Build history of the part. All positions in model axes, mm. Face numbers are marked on the shaded views. A direction names the side the tool comes from. Coordinates: 2 decimals unless noted, no trailing zeros. Order: outer loops, then holes, each group sorted by start corner. A loop starts at its lowest first (then second) coordinate and runs counter-clockwise, first axis right, second up. Notation, with made-up numbers: (87.25, 6.5) - (110.25, 6.5) arc R21 cw to (110.25, 22.5) - close; hole circle Ø11 at (-6, 79). An arc over 180 degrees is marked (long way). Return JSON: item names as keys, results as strings.
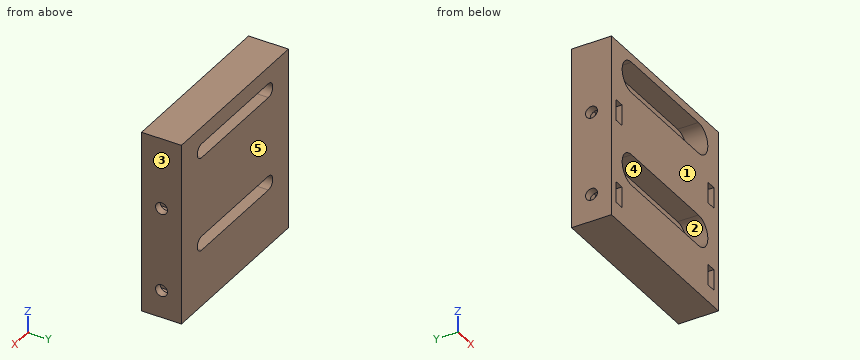
Autodesk Inventor part; units mm, degrees
ref_plane "YZ Plane" through (0, 0, 0) normal (1, 0, 0) x (0, 1, 0)
ref_plane "XZ Plane" through (0, 0, 0) normal (0, 1, 0) x (-1, 0, 0)
ref_plane "XY Plane" through (0, 0, 0) normal (0, 0, 1) x (1, 0, 0)
sketch "Sketch1" plane through (0, 0, 0) normal (0, 1, 0) x (-1, 0, 0)
  line L0 (-25.4, 20.32) -> (-25.4, -31.75)
  line L1 (-25.4, -31.75) -> (25.4, -31.75)
  line L2 (25.4, -31.75) -> (25.4, 20.32)
  line L3 (25.4, 31.75) -> (-25.4, -31.75) construction
  line L4 (-25.4, 31.75) -> (25.4, -31.75) construction
  line L5 (15.875, 13.4747) -> (-15.875, 13.4747) construction
  line L6 (15.875, 15.5067) -> (-15.875, 15.5067)
  line L7 (-15.875, 11.4427) -> (15.875, 11.4427)
  arc A0 (15.875, 11.4427) -> (15.875, 15.5067) centre (15.875, 13.4747) ccw
  arc A1 (-15.875, 15.5067) -> (-15.875, 11.4427) centre (-15.875, 13.4747) ccw
  line L8 (-15.875, -13.4747) -> (15.875, -13.4747) construction
  line L9 (-15.875, -15.5067) -> (15.875, -15.5067)
  line L10 (15.875, -11.4427) -> (-15.875, -11.4427)
  arc A2 (-15.875, -11.4427) -> (-15.875, -15.5067) centre (-15.875, -13.4747) ccw
  arc A3 (15.875, -15.5067) -> (15.875, -11.4427) centre (15.875, -13.4747) ccw
  line L11 (25.4, 20.32) -> (-25.4, 20.32)
  point P0 (0, 0)
  point P1 (0, 13.4747)
  point P2 (0, -13.4747)
  dimension "d0" = 50.8
  dimension "d2" = 26.9494
  dimension "d3" = 13.4747
  dimension "d4" = 26.9494
  dimension "d6" = 9.525
  dimension "d7" = 9.525
  dimension "d10" = 4.064
  dimension "d11" = 9.525
  dimension "d12" = 4.064
  dimension "d49" = 6.8453
extrude "Extrusion1" add sketch "Sketch1" along normal blind 11.43
sketch "Sketch3" plane through (0, 0, 0) normal (0, -1, 0) x (1, 0, 0)
  arc A0 (-15.875, -11.4427) -> (-15.875, -15.5067) centre (-15.875, -13.4747) ccw
  arc A1 (15.875, -15.5067) -> (15.875, -11.4427) centre (15.875, -13.4747) ccw
  line L0 (-15.875, -13.4747) -> (15.875, -13.4747) construction
  line L1 (-15.875, -17.9197) -> (15.875, -17.9197)
  line L2 (15.875, -9.0297) -> (-15.875, -9.0297)
  arc A2 (-15.875, -9.0297) -> (-15.875, -17.9197) centre (-15.875, -13.4747) ccw
  arc A3 (15.875, -17.9197) -> (15.875, -9.0297) centre (15.875, -13.4747) ccw
  arc A4 (-15.875, 15.5067) -> (-15.875, 11.4427) centre (-15.875, 13.4747) ccw
  arc A5 (15.875, 11.4427) -> (15.875, 15.5067) centre (15.875, 13.4747) ccw
  line L3 (-15.875, 13.4747) -> (15.875, 13.4747) construction
  line L4 (-15.875, 9.0297) -> (15.875, 9.0297)
  line L5 (15.875, 17.9197) -> (-15.875, 17.9197)
  arc A6 (-15.875, 17.9197) -> (-15.875, 9.0297) centre (-15.875, 13.4747) ccw
  arc A7 (15.875, 9.0297) -> (15.875, 17.9197) centre (15.875, 13.4747) ccw
  point P0 (0, 0)
  point P1 (0, -13.4747)
  point P2 (0, 13.4747)
  dimension "d19" = 8.89
  dimension "d20" = 8.89
extrude "Extrusion3" cut sketch "Sketch3" against normal blind 5.9436
ref_plane "Work Plane2" through (-20.4, 0, -31.75) normal (-1, 0, 0) x (0, 0, 1)
sketch "Sketch5" plane through (-20.4, 0, -31.75) normal (-1, 0, 0) x (0, 0, 1)
  circle A0 centre (31.75, 5.715) radius 3.45 construction
  line L0 (52.07, 0) -> (0, 0)
  line L1 (52.07, 11.43) -> (0, 11.43)
  line L2 (0, 0) -> (0, 11.43)
  line L3 (28.7622, 0) -> (28.7622, 7.44)
  line L4 (28.7622, 7.44) -> (31.75, 9.165)
  line L5 (31.75, 9.165) -> (34.7378, 7.44)
  line L6 (34.7378, 7.44) -> (34.7378, 0)
  line L7 (28.7622, 0) -> (34.7378, 0)
  line L8 (13.8303, 0) -> (13.8303, 5.9436) construction
  line L9 (49.6697, 0) -> (49.6697, 5.9436) construction
  circle A1 centre (7.8403, 5.715) radius 3.45 construction
  line L10 (4.8525, 0) -> (4.8525, 7.44)
  line L11 (4.8525, 7.44) -> (7.8403, 9.165)
  line L12 (7.8403, 9.165) -> (10.8281, 7.44)
  line L13 (10.8281, 7.44) -> (10.8281, 0)
  line L14 (4.8525, 0) -> (10.8281, 0)
  circle A2 centre (7.8403, 5.715) radius 1.7
  circle A3 centre (31.75, 5.715) radius 1.7
  point P0 (31.75, 0)
  dimension "d24" = 6.9
  dimension "d26" = 5.715
  dimension "d29" = 6.9
  dimension "d31" = 5.99
  dimension "d33" = 5.715
  dimension "d37" = 3.4
  dimension "d38" = 3.4
  dimension "d48" = 31.75
extrude "Extrusion4" cut sketch "Sketch5" along normal blind 2.8 contours L0 L10 L11 L12 L13 | L0 L3 L4 L5 L6 | A2 | A3
sketch "Sketch6" plane through (-25.4, 0, -31.75) normal (-1, 0, 0) x (0, 0, 1)
  circle A0 centre (7.8403, 5.715) radius 1.7
  circle A1 centre (31.75, 5.715) radius 1.7
  line L0 (13.8303, 0) -> (13.8303, 5.9436)
  line L1 (63.5, 0) -> (63.5, 11.43)
  line L2 (49.6697, 0) -> (49.6697, 5.9436)
  point P0 (31.75, 0)
  dimension "d40" = 3.4
  dimension "d41" = 3.4
  dimension "d43" = 5.99
extrude "Extrusion5" cut sketch "Sketch6" against normal blind 6
ref_plane "Work Plane3" through (0, 0, -31.75) normal (-1, 0, 0) x (0, 0, 1)
mirror "Mirror1" about plane through (0, 0, -31.75) normal (-1, 0, 0) of "Extrusion4"
mirror "Mirror2" about plane through (0, 0, -31.75) normal (-1, 0, 0) of "Extrusion5"
sketch "Sketch7" plane through (0, 0, 0) normal (0, -1, 0) x (1, 0, 0)
  point P0 (0, 0)
equation "\"d4\" = d2"
equation "\"d26\" = 0.5 * d25"
equation "\"d33\" = d26"
equation "\"d43\" = d31"
properties part number "driven wheel mount to xrail"
1. Mould opens along X. For the marked faces 1, 2 and 3 say: pulls with the +X half, pulls with the -X half, needs draft (parallel to the pull), parting line crosses it, or undercut.
Check values:
{"face 1": "needs draft", "face 2": "undercut", "face 3": "pulls with the +X half"}
2. Cut at A-A on x = -6. Give the cut face in (y, z).
Check values:
{"outline": "(0, -31.75) - (11.43, -31.75) - (11.43, -15.51) - (5.94, -15.51) - (5.94, -17.92) - (0, -17.92) - close; (0, -9.03) - (5.94, -9.03) - (5.94, -11.44) - (11.43, -11.44) - (11.43, 11.44) - (5.94, 11.44) - (5.94, 9.03) - (0, 9.03) - close; (0, 17.92) - (5.94, 17.92) - (5.94, 15.51) - (11.43, 15.51) - (11.43, 20.32) - (0, 20.32) - close"}
3. Tool access for the marked faces 4 and 5: list every direction of +Z, -Z, +X, -X, +Y, -Y with a clear straight run to the whole face (end or side of a thin tool).
Check values:
{"face 4": "-Y", "face 5": "+Z, -Z, +X, -X, +Y"}
4. Probe L1, parallel to Z at x = 4.5, y = 9.75; L2, parallel to X at y = 0.75, z = 0.5; L3, parallel to Z at x = 4, y = 1.5. List the from-to ranges inside material, lowest first.
Check values:
{"L1": "-31.75 to -15.51, -11.44 to 11.44, 15.51 to 20.32", "L2": "-25.4 to -23.2, -20.4 to 20.4, 23.2 to 25.4", "L3": "-31.75 to -17.92, -9.03 to 9.03, 17.92 to 20.32"}
5. Drop flat-ended pins along their axis: pin 1 (3 mm diameter, centred on x = 10.5, z = -25.5, fed in from -Y); pin 2 (4.5 mm diameter, centred on x = 5.5, z = -14.5, fed in from -Y). Give the stop position or say it passes through.
Check values:
{"pin 1": "y = 0", "pin 2": "y = 5.94"}
6. Cut at C-C on z = -13. Give the cut face in (x, y), plus the area to 3 significant figures.
Check values:
{"outline": "(-25.4, 0) - (-20.29, 0) - (-20.29, 5.94) - (-17.85, 5.94) - (-17.85, 11.43) - (-25.4, 11.43) - close; (17.85, 5.94) - (20.29, 5.94) - (20.29, 0) - (25.4, 0) - (25.4, 11.43) - (17.85, 11.43) - close", "area": "144 mm²"}
7. Cut at B-B on y = 3. State how many separate pieces and enclosed holes the cut face has, plus the area to 3 significant figures.
Check values:
{"separate pieces": "1", "enclosed holes": "6", "area": "1,890 mm²"}
